```python
from build123d import *

# Parameters (mm, degrees)
F0_R     = 6.35
F1_DEPTH = 6.35
F2_R     = 12.7
F2_R_2   = 6.35
F3_DEPTH = 19.05


with BuildPart() as f1:
    # F0 (on Top) → F1 (new body)
    with BuildSketch(Plane.XY):
        with BuildLine():
            Line((31.75, 0), (0, 0))
            ThreePointArc((0, 0), (-12.7, -12.7), (0, -25.4))
            Line((0, -25.4), (19.05, -25.4))
            Line((19.05, -25.4), (31.75, -12.7))
            Line((31.75, -12.7), (31.75, 0))
        make_face()
        with Locations((0, -12.7)):
            Circle(F0_R, mode=Mode.SUBTRACT)
    extrude(amount=F1_DEPTH)

    # F2 (on face) → F3 (join)
    with BuildSketch(Plane.XY.offset(6.35)):
        with Locations((0, -12.7)):
            Circle(F2_R)
        with Locations((0, -12.7)):
            Circle(F2_R_2, mode=Mode.SUBTRACT)
    extrude(amount=F3_DEPTH)


solid = f1.part
```
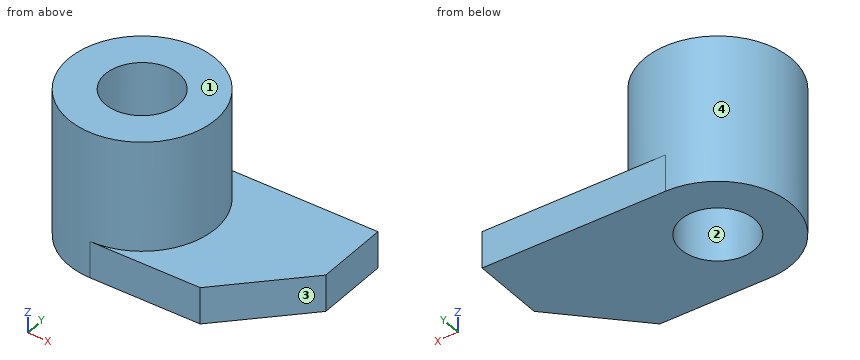
For this review, take the finished solid that the model builds, in its own axes (mm). Face numbers are marked on the shaded views. Coordinates: 2 decimals unless noted, no trailing zeros. Order: outer loops, then holes, each group sorted by start corner. A loop starts at its lowest first (then second) coordinate and runs counter-clockwise, first axis right, second up. Notation, with made-up numbers: (25, -4.5) -> (59, -4.5) arc R20 ccw to (59, 26.5) -> close; hole circle Ø9 at (81.25, -35). An arc over 180 degrees is marked (long way). Use CSV: the item, a comma, the result in double quotes. Start each with the question number.
Item 1: We need section B-B, the plane z = 5.25. Give the boundary of the cut face in (x, y).
Item 2: Wall thickness on probe 1 along Y at (x, z) = (0, 19.25); probe 2 along Z at (x, y) = (16, -5.5); probe 3 along X at (y, z) = (-16, 22.5): over which ranges is each line inside the solid? List them lowest first.
Item 3: Insertion check: pin 1 (3 mm diameter, centred on y = -17, z = 19.5, fed in from -X); pin 2 (8 mm diameter, centred on y = -19, z = 19.5, fed in from -X); pin 3 (1 mm diameter, centred on y = -8, z = 12.5, fed in from -X); pin 4 (5 mm diameter, centred on x = -2, z = 14.5, fed in from -Y). Each pin has a flat end and moves straight along its axis. Give the tip position at first contact, or say it passes through.
Item 4: We need section D-D, the plane x = 7. Give the boundary of the cut face in (y, z), then the cut area to 3 significant figures.
Item 5: We need section A-A, the plane x = -5. Give the boundary of the cut face in (y, z), then the cut area to 3 significant figures.
Item 6: We need section C-C, the plane y = -14.25. Give the boundary of the cut face in (x, z).
Item 7: Draft analysis for pull direction X (two halves, no side actions). For the marked faces 1, 2, 3 and 4, state which applies: pulls with the +X half, pulls with the -X half, needs draft (parallel to the pull), parting line crosses it, or undercut.
Derived:
1,outline,"(0, -25.4) -> (19.05, -25.4) -> (31.75, -12.7) -> (31.75, 0) -> (0, 0) arc R12.7 ccw to start; hole circle Ø12.7 at (0, -12.7)"
2,probe 1,"y = -25.4 to -19.05, -6.35 to 0"
2,probe 2,"z = 0 to 6.35"
2,probe 3,"x = -12.26 to -5.43, 5.43 to 12.26"
3,pin 1,"stops at x = -12.39"
3,pin 2,"stops at x = -12.49"
3,pin 3,"stops at x = -11.99"
3,pin 4,"stops at y = -25.4"
4,outline,"(-25.4, 0) -> (0, 0) -> (0, 6.35) -> (-2.1, 6.35) -> (-2.1, 25.4) -> (-23.3, 25.4) -> (-23.3, 6.35) -> (-25.4, 6.35) -> close"
4,area,"565 mm^2"
5,outline,"(-24.37, 0) -> (-16.61, 0) -> (-16.61, 25.4) -> (-24.37, 25.4) -> close; (-8.79, 0) -> (-1.03, 0) -> (-1.03, 25.4) -> (-8.79, 25.4) -> close"
5,area,"394 mm^2"
6,outline,"(-12.61, 0) -> (-6.16, 0) -> (-6.16, 25.4) -> (-12.61, 25.4) -> close; (6.16, 0) -> (30.2, 0) -> (30.2, 6.35) -> (12.61, 6.35) -> (12.61, 25.4) -> (6.16, 25.4) -> close"
7,face 1,"needs draft"
7,face 2,"undercut"
7,face 3,"pulls with the +X half"
7,face 4,"parting line crosses it"
